Design review of the part built by this model. Coordinates are the model's own, in mm. Give positions to 0.01 mm unless a question says otherwise; leave off trailing zeros. Loops run counter-clockwise (first coordinate to the right, second up) from the corner with the lowest first, then second, coordinate; pieces in that order, holes last. Notation, with made-up numbers: (58, 37.25) -> (66, 37.25) arc R18 ccw to (66, 54.25) -> close; hole circle Ø8 at (17.5, 77.25). An arc over 180 degrees is marked (long way). Answer in a Markdown table with one row per item. Add a question column.
(1) For pin 1 (2.5 mm diameter, centred on x = -72, y = 98, fed in from -Z); pin 2 (10 mm diameter, centred on x = 121, y = 93, fed in from -Z), all flat-tipped, find the tip position at first contact; note any pin that passes through.
(2) Consider section A-A on x = -12. Write out the cut boundary in (y, z).
(3) Draft analysis for pull direction Y (two halves, no side actions). For faces 1 (the flat face through (3, 99, 4)), 2 (the flat face through (3, 55, 12)), 3 (the flat face through (3, 108, 6)), state which applies: +Y half, -Y half, draft (parallel to the pull), parting line (faces both ways), or undercut.
(4) For line 1 (Y direction, x = 42.5, z = 3.5); line 2 (Z direction, x = -130.5, y = 100.5), list the stretches that pass through material, from the lowest coordinate up.
from build123d import *

# Parameters (mm, degrees)
F1_DEPTH = 200
F2_R     = 1


with BuildPart() as f1:
    # F0 (on Right) → F1 (new body, symmetric)
    with BuildSketch(Plane.YZ):
        Polygon((108, 12), (0, 12), (0, 0), (94.5, 0), (94.5, 4), (103, 4), (103, 0), (108, 0), align=None)
    extrude(amount=F1_DEPTH, both=True)

    # F2
    f2_edges = [f1.edges().sort_by_distance(p)[0] for p in [
        (200, 0, 6),
        (200, 108, 6),
        (-200, 108, 6),
        (-200, 0, 6),
    ]]
    fillet(f2_edges, radius=F2_R)


solid = f1.part
Values follow:
| question | item | result |
|---|---|---|
| 1 | pin 1 | z = 4 |
| 1 | pin 2 | z = 0 |
| 2 | outline | (0, 0) -> (94.5, 0) -> (94.5, 4) -> (103, 4) -> (103, 0) -> (108, 0) -> (108, 12) -> (0, 12) -> close |
| 3 | face 1 | undercut |
| 3 | face 2 | draft |
| 3 | face 3 | +Y half |
| 4 | line 1 | 0 to 94.5, 103 to 108 |
| 4 | line 2 | 4 to 12 |
